Verification items for the finished model (mm, model axes). A direction names the side the tool comes from. Round coordinates to 2 decimals unless told otherwise and drop trailing zeros. Order: outer loops, then holes, each group sorted by start corner. A loop starts at its lowest first (then second) coordinate and runs counter-clockwise, first axis right, second up. Notation, with made-up numbers: (-23.75, 32.25) -> (16.25, 32.25) arc R26 ccw to (16.25, 47.25) -> close; hole circle Ø8 at (-33.5, -38). An arc over 180 degrees is marked (long way). Put each result on its own line as item: value.
from build123d import *

# Parameters (mm, degrees)
CROQUIS1_R              = 3
SALIENTE_EXTRUIR1_DEPTH = 3


with BuildPart() as part:
    # Croquis1 → Saliente-Extruir1 (new body)
    with BuildSketch(Plane(origin=(0, 0, 0), x_dir=(1, 0, 0), z_dir=(0, 1, 0))):
        Polygon((0, 3), (110, 3), (110, 12.5), (107, 12.5), (107, 20), (107, 27.5), (110, 27.5), (110, 37), (110, 140), (89.5, 140), (20.5, 140), (0, 140), (0, 50), (0, 35), (3, 35), (3, 20), (3, 15), (0, 15), align=None)
        with Locations(Location((10.25, 60.5, 0), (0, 0, 270))):
            Circle(CROQUIS1_R, mode=Mode.SUBTRACT)
        with Locations(Location((99.75, 60.5, 0), (0, 0, 270))):
            Circle(CROQUIS1_R, mode=Mode.SUBTRACT)
        with Locations(Location((10.25, 99.5, 0), (0, 0, 270))):
            Circle(CROQUIS1_R, mode=Mode.SUBTRACT)
        Polygon((92.5, 37), (89.5, 37), (20.5, 37), (17.5, 37), (17.5, 40), (20.5, 40), (20.5, 130), (89.5, 130), (89.5, 40), (92.5, 40), align=None, mode=Mode.SUBTRACT)
        with Locations(Location((99.75, 99.5, 0), (0, 0, 270))):
            Circle(CROQUIS1_R, mode=Mode.SUBTRACT)
    extrude(amount=SALIENTE_EXTRUIR1_DEPTH)


solid = part.part
Item 1: Section check A-A on x = 99.75. Record the boundary of the cut face in (y, z).
Check sheet entries:
outline: (0, -140) -> (3, -140) -> (3, -102.5) -> (0, -102.5) -> close; (0, -96.5) -> (3, -96.5) -> (3, -63.5) -> (0, -63.5) -> close; (0, -57.5) -> (3, -57.5) -> (3, -3) -> (0, -3) -> close
Item 2: Section check B-B on x = 50.5. Record the boundary of the cut face in (y, z), then the cut area to 3 significant figures.
Check sheet entries:
outline: (0, -140) -> (3, -140) -> (3, -130) -> (0, -130) -> close; (0, -37) -> (3, -37) -> (3, -3) -> (0, -3) -> close
area: 132 mm^2
Item 3: Section check D-D on z = -99.5. Record the boundary of the cut face in (x, y).
Check sheet entries:
outline: (0, 0) -> (7.25, 0) -> (7.25, 3) -> (0, 3) -> close; (13.25, 0) -> (20.5, 0) -> (20.5, 3) -> (13.25, 3) -> close; (89.5, 0) -> (96.75, 0) -> (96.75, 3) -> (89.5, 3) -> close; (102.75, 0) -> (110, 0) -> (110, 3) -> (102.75, 3) -> close
Item 4: Gauge pin test, flat end, axial feed: pin 1 Ø1.5 at (y, z) = (1, -20.5) entering from -X. Record the tip position at first contact, or that the pin passes through.
Check sheet entries:
pin 1: stops at x = 3
Item 5: Section check C-C on z = -85.5. Record the boundary of the cut face in (x, y).
Check sheet entries:
outline: (0, 0) -> (20.5, 0) -> (20.5, 3) -> (0, 3) -> close; (89.5, 0) -> (110, 0) -> (110, 3) -> (89.5, 3) -> close
Item 6: Release check for a two-part mould opening along X. For faces 4 (the flat face through (18, 3, -72)), 5 (the flat face through (89.5, 1, -86)), 6 (the flat face through (92.5, 1, -39)), 7 (the flat face through (0, 1, -9)) record: +X half, -X half, draft (parallel to the pull), parting line (faces both ways), or undercut.
Check sheet entries:
face 4: draft
face 5: undercut
face 6: undercut
face 7: -X half
Item 7: Tool access check on faces 1 (the flat face through (2, 1, -15)), 2 (the flat face through (107, 1, -20)), 3 (the flat face through (55, 1, -130)). Record the directions out of +Z, -Z, +X, -X, +Y, -Y that give a thin tool (end or side, any length) a straight path to the whole face; none if there is none.
Check sheet entries:
face 1: -X, +Y, -Y
face 2: +X, +Y, -Y
face 3: +Y, -Y
Item 8: Material ranges on L1, parallel to X at y = 2.3, z = -60.5; L2, parallel to Z at x = 31.5, y = 2; L3, parallel to X at y = 2.2, z = -126.5, recorded low to high. Write a range as [from, to].
Check sheet entries:
L1: x = [0, 7.25], [13.25, 20.5], [89.5, 96.75], [102.75, 110]
L2: z = [-140, -130], [-37, -3]
L3: x = [0, 20.5], [89.5, 110]
